```python
from build123d import *

# Parameters (mm, degrees)
CROQUIS1_W              = 16
CROQUIS1_H              = 2
SALIENTE_EXTRUIR1_DEPTH = 13
CORTAR_EXTRUIR1_DEPTH   = 21.712315177


with BuildPart() as part:
    # Croquis1 → Saliente-Extruir1 (new body)
    with BuildSketch(Plane(origin=(0, 0, 0), x_dir=(1, 0, 0), z_dir=(0, 1, 0))):
        with Locations((8, 1)):
            Rectangle(CROQUIS1_W, CROQUIS1_H)
    extrude(amount=SALIENTE_EXTRUIR1_DEPTH)

    # Croquis2 → Cortar-Extruir1 (cut, through all)
    with BuildSketch(Plane(origin=(0, 0, -2), x_dir=(-1, 0, 0), z_dir=(0, 0, -1))):
        with BuildLine():
            Line((-4, 6.5), (-4, 13))
            Line((-4, 13), (-12, 13))
            Line((-12, 13), (-12, 6.5))
            ThreePointArc((-12, 6.5), (-8, 2.5), (-4, 6.5))
        make_face()
    extrude(amount=-CORTAR_EXTRUIR1_DEPTH, mode=Mode.SUBTRACT)


solid = part.part
```
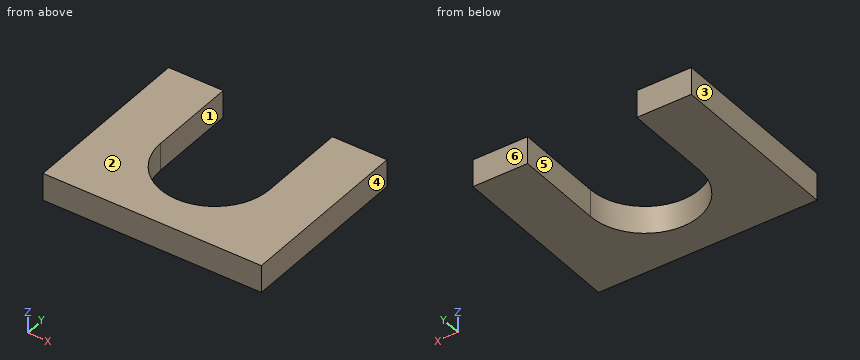
Model file for the job. Use its own axes, mm. Face numbers are marked on the shaded views. A direction names the side the tool comes from. Give positions to 0.01 mm unless a question says otherwise; leave off trailing zeros. Order: outer loops, then holes, each group sorted by start corner. A loop starts at its lowest first (then second) coordinate and runs counter-clockwise, first axis right, second up.
1) Saw through at B-B, the plane z = -1.6. Write the cut outline in (x, y).
2) 3-axis set-ups, long thin cutter, end or side, ignore diameter. For the marked faces 5 and 6: which of +Z, -Z, +X, -X, +Y, -Y reach the whole face in a straight line?
3) Wall check: probe 1 along X at (y, z) = (9.75, -0.4); probe 2 along Y at (x, z) = (8, -1.15); probe 3 along X at (y, z) = (4.5, -1.7). Give the ranges that are in metal, low to high.
4) Saw through at A-A, the plane y = 6.75. Write the cut outline in (x, z), then the cut area to 3 significant figures.
5) Mould opens along X. For the marked faces 1, 2, 3 and 4 say: +X half, -X half, draft (parallel to the pull), parting line (faces both ways), or undercut.
6) Saw through at C-C, the plane x = 8. Write the cut outline in (y, z).
Computed:
1. outline: (0, 0) - (16, 0) - (16, 13) - (12, 13) - (12, 6.5) arc R4 cw to (4, 6.5) - (4, 13) - (0, 13) - close
2. face 5: +Z, -Z, +Y
2. face 6: +Z, -Z, +X, -X, +Y
3. probe 1: x = 0 to 4, 12 to 16
3. probe 2: y = 0 to 2.5
3. probe 3: x = 0 to 4.54, 11.46 to 16
4. outline: (0, -2) - (4, -2) - (4, 0) - (0, 0) - close; (12, -2) - (16, -2) - (16, 0) - (12, 0) - close
4. area: 16.0 mm2
5. face 1: undercut
5. face 2: draft
5. face 3: -X half
5. face 4: +X half
6. outline: (0, -2) - (2.5, -2) - (2.5, 0) - (0, 0) - close
